Design review of the part built by this model. Coordinates are the model's own, in mm. A direction names the side the tool comes from. Coordinates: 2 decimals unless noted, no trailing zeros. Write each loop counter-clockwise with the first axis right and the second up, starting at its lowest first coordinate (ties: lowest second). Pieces come first, ordered by that corner, then holes. Notation, with made-up numbers: (83, 15) - (123, 15) arc R22 cw to (123, 26) - close; hole circle Ø4 at (-19.5, -10.5). An arc over 180 degrees is marked (long way). Use a Markdown table: item, result.
from build123d import *

# Parameters (mm, degrees)
MODEL_R             = 3.6
MODEL_R_2           = 1.3
BOSS_EXTRUDE1_DEPTH = 3


with BuildPart() as part:
    # Model → Boss-Extrude1 (new body)
    with BuildSketch(Plane.XY):
        with BuildLine():
            Line((58.068440008, 48.533872703), (46.830105606, 35.365817257))
            ThreePointArc((46.830105606, 35.365817257), (46.085714126, 33.921588349), (45.843713156, 32.314929909))
            ThreePointArc((45.843713156, 32.314929909), (36.762881301, 28.086852553), (39.424151137, 37.743756206))
            ThreePointArc((39.424151137, 37.743756206), (41.006745997, 38.235421473), (42.341707312, 39.217368271))
            Line((42.341707312, 39.217368271), (53.580041714, 52.385423717))
            ThreePointArc((53.580041714, 52.385423717), (57.749130002, 52.715057779), (58.078764064, 48.54596949))
            Line((58.078764064, 48.54596949), (58.068440008, 48.533872703))
        make_face()
        with Locations((40.325895646, 32.300100558)):
            Circle(MODEL_R, mode=Mode.SUBTRACT)
        with Locations((55.829402889, 50.465696604)):
            Circle(MODEL_R_2, mode=Mode.SUBTRACT)
        with BuildLine():
            Line((47.314287018, 39.487196923), (50.544132712, 43.310523772))
            ThreePointArc((50.544132712, 43.310523772), (50.470318272, 44.19097138), (49.589870666, 44.117156913))
            Line((49.589870666, 44.117156913), (46.321463386, 40.326423493))
            ThreePointArc((46.321463386, 40.326423493), (46.398261906, 39.41039838), (47.314287018, 39.487196923))
        make_face(mode=Mode.SUBTRACT)
    extrude(amount=BOSS_EXTRUDE1_DEPTH)


solid = part.part
(1) Draft analysis for pull direction X (two halves, no side actions). For faces 3 (the cylindrical face through (40.986, 38.225, 1.479)), 4 (the flat face through (46, 41, 3)), 5 (the cylindrical face through (36.73, 32.46, 1.48)), 6 (the cylindrical face through (36.899, 27.976, 1.479)), state which applies: +X half, -X half, draft (parallel to the pull), parting line (faces both ways), or undercut.
Determined:
| item | result |
|---|---|
| face 3 | -X half |
| face 4 | draft |
| face 5 | undercut |
| face 6 | parting line |
(2) Take a section at C-C on z = 1.1. Write out the cut boundary in (x, y).
Determined:
| item | result |
|---|---|
| outline | (39.42, 37.74) arc R5.52 ccw (long way) to (45.84, 32.31) arc R5 cw to (46.83, 35.37) - (58.08, 48.55) arc R2.96 ccw to (53.58, 52.39) - (42.34, 39.22) arc R5 cw to start; hole circle Ø7.2 at (40.33, 32.3); hole (46.32, 40.33) arc R0.65 ccw to (47.31, 39.49) - (50.54, 43.31) arc R0.62 ccw to (49.59, 44.12) - close; hole circle Ø2.6 at (55.83, 50.47) |
(3) For L1, parallel to Y at x = 50, z = 1.75 (3 decimals); L2, parallel to X at y = 31, z = 0.8; L3, parallel to X at y = 34, z = 1.5, list the stretches that pass through material, from the lowest coordinate up. Write a range as from..to.
Determined:
| item | result |
|---|---|
| L1 | 39.08..42.666, 44.335..48.191 |
| L2 | 34.96..36.97, 43.68..45.69 |
| L3 | 35.08..37.15, 43.5..46.11 |
(4) Take a section at D-D on y = 37. Write out the cut boundary in (x, z).
Determined:
| item | result |
|---|---|
| outline | (37.43, 0) - (48.22, 0) - (48.22, 3) - (37.43, 3) - close |
(5) Take a section at A-A on x = 56. Write out the cut boundary in (y, z), and give its area (3 significant figures).
Determined:
| item | result |
|---|---|
| outline | (46.11, 0) - (49.18, 0) - (49.18, 3) - (46.11, 3) - close; (51.75, 0) - (53.42, 0) - (53.42, 3) - (51.75, 3) - close |
| area | 14.2 mm2 |
(6) Machinability: for faces 1 (the flat face through (47.98, 42.25, 1.48)), 2 (the flat face through (46, 41, 0)), which of the approach directions +Z, -Z, +X, -X, +Y, -Y give a long, thin tool a straight path to every point of the face, cutting with its end or side? Answer none if there is none.
Determined:
| item | result |
|---|---|
| face 1 | +Z, -Z |
| face 2 | -Z, +X, -X, +Y, -Y |
(7) Take a section at B-B on y = 30.5. Write out the cut boundary in (x, z), and give its area (3 significant figures).
Determined:
| item | result |
|---|---|
| outline | (35.11, 0) - (37.21, 0) - (37.21, 3) - (35.11, 3) - close; (43.44, 0) - (45.54, 0) - (45.54, 3) - (43.44, 3) - close |
| area | 12.6 mm2 |
